Geometry check sheet. Reference: drawing and pictorial views, mm from the part's lowest x, y, z. A direction names the side the tool comes from. Round coordinates to 2 decimals unless told otherwise and drop trailing zeros. Write each loop counter-clockwise with the first axis right and the second up, starting at its lowest first coordinate (ties: lowest second). Pieces come first, ordered by that corner, then holes. Notation, with made-up numbers: (42, 49.5) - (60, 49.5) arc R16 ccw to (60, 64.5) - close; hole circle Ø3 at (51.25, -16.75). An arc over 180 degrees is marked (long way). Return JSON: item names as keys, results as strings.
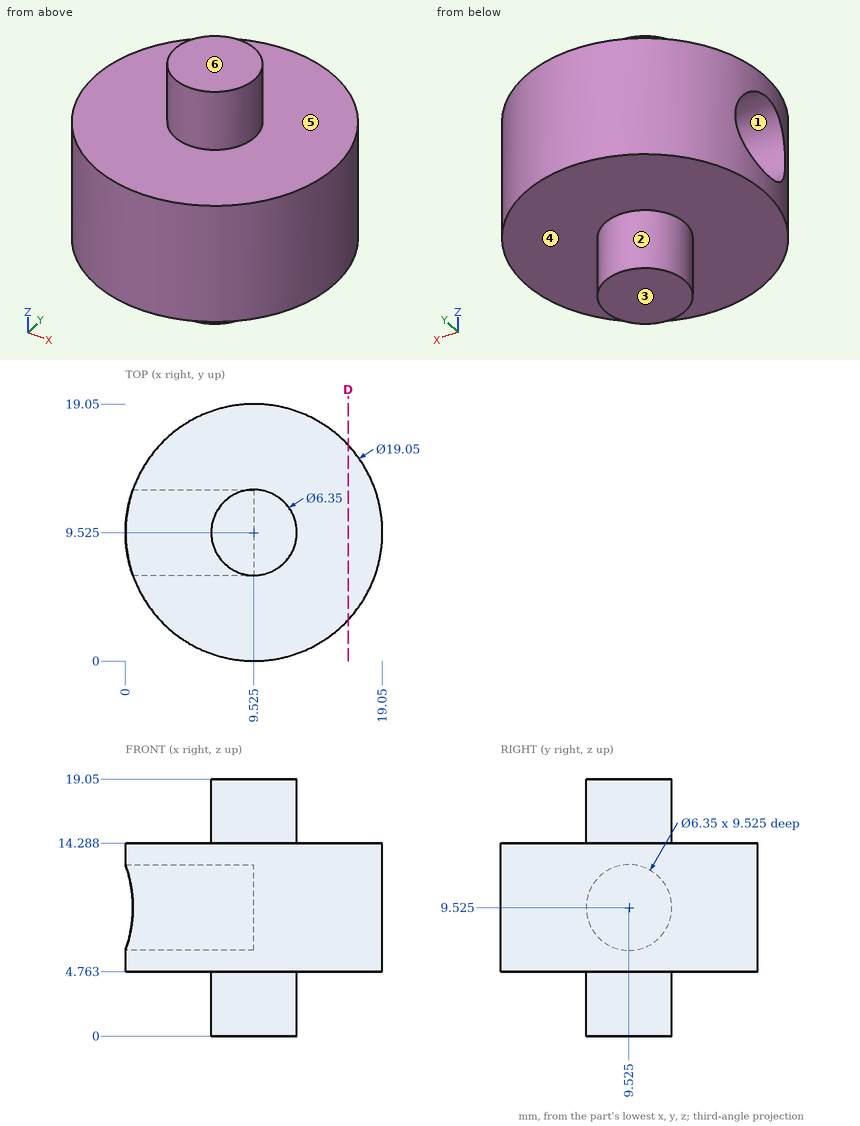
(1) Section check D-D, the plane x = 16.5. Enter the section's corners in (y, z).
Response values:
{"outline": "(3.04, 4.76) - (16.01, 4.76) - (16.01, 14.29) - (3.04, 14.29) - close"}
(2) Material ranges on line 1 along Z through (x, y) = (3, 9.5); line 2 along Z through (x, y) = (5.75, 17.5); line 3 along Y through (x, z) = (4.75, 8.5) (1 decimal), recorded low to high. Write a range as [from, to].
Response values:
{"line 1": "z = [4.76, 6.35], [12.7, 14.29]", "line 2": "z = [4.76, 14.29]", "line 3": "y = [1.3, 6.5], [12.5, 17.8]"}
(3) Access from +Z, -Z, +X, -X, +Y, -Y to the whole of each face (thin tool, end or side, straight path). Record for the marked faces 4, 5 and 6.
Response values:
{"face 4": "-Z", "face 5": "+Z", "face 6": "+Z, +X, -X, +Y, -Y"}
(4) Release check for a two-part mould opening along Z. For the marked faces 1, 2 and 3 record: pulls with the +Z half, pulls with the -Z half, needs draft (parallel to the pull), parting line crosses it, or undercut.
Response values:
{"face 1": "undercut", "face 2": "needs draft", "face 3": "pulls with the -Z half"}
(5) Gauge pin test, flat ends, axial feed: pin 1 (8 mm diameter, centred on y = 15, z = 8.5, fed in from -X); pin 2 (4 mm diameter, centred on x = 12.5, z = 13, fed in from -Y); pin 3 (1.9 mm diameter, centred on y = 8.5, z = 11, fed in from -X) (1 decimal); pin 4 (3 mm diameter, centred on y = 10.5, z = 6.5, fed in from -X). Record the tip position at first contact, or that the pin passes through.
Response values:
{"pin 1": "stops at x = 0.17", "pin 2": "stops at y = 0.05", "pin 3": "stops at x = 9.5", "pin 4": "stops at x = 0"}
